```python
from build123d import *

# Parameters (mm, degrees)
SKETCH_1_R          = 10
SKETCH_1_R_2        = 9.5
EXTRUDE_1_DEPTH     = 10
SKETCH_2_R          = 1.65
CUT_EXTRUDE_1_DEPTH = 18.320508076
SKETCH_3_W          = 5
SKETCH_3_H          = 20.666812771
CUT_EXTRUDE_2_DEPTH = 18.320508249


with BuildPart() as part:
    # 草图1 → 凸台-拉伸1 (new body)
    with BuildSketch(Plane.XY):
        Circle(SKETCH_1_R)
        Circle(SKETCH_1_R_2, mode=Mode.SUBTRACT)
    extrude(amount=EXTRUDE_1_DEPTH)

    # 草图2 → 切除-拉伸1 (cut, through all)
    with BuildSketch(Plane(origin=(0, 0, 0), x_dir=(1, 0, 0), z_dir=(0, 1, 0))):
        with Locations(Location((0, -4.882407133, 0), (0, 0, 90))):
            Circle(SKETCH_2_R)
    extrude(amount=CUT_EXTRUDE_1_DEPTH, mode=Mode.SUBTRACT)

    # 草图3 → 切除-拉伸2 (cut, through all)
    with BuildSketch(Plane(origin=(0, 0, 0), x_dir=(1, 0, 0), z_dir=(0, 1, 0))):
        with Locations((0, -4.882407133)):
            Rectangle(SKETCH_3_W, SKETCH_3_H)
    extrude(amount=-CUT_EXTRUDE_2_DEPTH, mode=Mode.SUBTRACT)


solid = part.part
```
The listing builds one solid part. Answer for the finished solid, in the listing's coordinates (mm). Coordinates: 2 decimals unless noted, no trailing zeros. Write each loop counter-clockwise with the first axis right and the second up, starting at its lowest first coordinate (ties: lowest second). Pieces come first, ordered by that corner, then holes.
Q1. Section A-A, the plane x = 0 is taken. Write down the section's boundary in (y, z), then the cut area to 3 significant figures.
Returned:
outline: (9.5, 0) - (10, 0) - (10, 3.23) - (9.5, 3.23) - close; (9.5, 6.53) - (10, 6.53) - (10, 10) - (9.5, 10) - close
area: 3.35 mm2
Q2. Section C-C, the plane z = 7.25 is taken. Write down the section's boundary in (x, y).
Returned:
outline: (-2.5, -9.68) - (-2.5, -9.17) arc R9.5 cw (long way) to (2.5, -9.17) - (2.5, -9.68) arc R10 ccw (long way) to start
Q3. Find the intervals of material crossed by line 1 along X through (y, z) = (0, 7); line 2 along X through (y, z) = (-6, 4.5); line 3 along Y through (x, z) = (7, 4), in increasing order.
Returned:
line 1: x = -10 to -9.5, 9.5 to 10
line 2: x = -8 to -7.37, 7.37 to 8
line 3: y = -7.14 to -6.42, 6.42 to 7.14
Q4. Section B-B, the plane y = 1 is taken. Write down the section's boundary in (x, z), then the cut area to 3 significant figures.
Returned:
outline: (-9.95, 0) - (-9.45, 0) - (-9.45, 10) - (-9.95, 10) - close; (9.45, 0) - (9.95, 0) - (9.95, 10) - (9.45, 10) - close
area: 10.1 mm2
Q5. The mould has two halves that part along X. Classify faces 1 (the flat face through (4, 9, 10)), 2 (the cylindrical face through (1.464, 9.675, 4.121)): released by +X, released by -X, zero draft, split by the parting line, or undercut.
Returned:
face 1: zero draft
face 2: undercut
Q6. Given P1, Ø3, axis at y = -6.5, z = 1.5, coming from the -X side; P2, Ø4, axis at x = 0, z = 4.88, coming from the -Y side; P3, Ø2, axis at x = -5.5, z = 3, coming from the -Y side, each flat-ended and moving along its own axis, determine where each tip first touches the part or whether it passes through.
Returned:
P1: stops at x = -8.66
P2: stops at y = 9.29
P3: stops at y = -8.93
